from build123d import *

# Parameters (mm, degrees)
F0_W          = 57.15
F0_H          = 57.15
F0_W_2        = 51.054
F0_H_2        = 51.054
F1_DEPTH      = 304.8
F2_R          = 3.048
F3_R          = 6.35
F5_DEPTH      = 28.576
F5_DEPTH_BACK = 28.576
F7_DEPTH      = 28.576
F7_DEPTH_BACK = 28.576


with BuildPart() as f1:
    # F0 (on Top) → F1 (new body)
    with BuildSketch(Plane.XY):
        Rectangle(F0_W, F0_H)
        Rectangle(F0_W_2, F0_H_2, mode=Mode.SUBTRACT)
    extrude(amount=F1_DEPTH)

    # F2
    f2_edges = [f1.edges().sort_by_distance(p)[0] for p in [
        (25.527, 25.527, 152.4),
        (-25.527, 25.527, 152.4),
        (-25.527, -25.527, 152.4),
        (25.527, -25.527, 152.4),
    ]]
    fillet(f2_edges, radius=F2_R)

    # F3
    f3_edges = [f1.edges().sort_by_distance(p)[0] for p in [
        (-28.575, 28.575, 152.4),
        (-28.575, -28.575, 152.4),
        (28.575, -28.575, 152.4),
        (28.575, 28.575, 152.4),
    ]]
    fillet(f3_edges, radius=F3_R)

    # F4 (on Front) → F5 (cut, two sides)
    with BuildSketch(Plane.XZ) as f5_sk:
        Polygon((-28.575, 247.65), (28.575, 304.8), (-28.575, 304.8), align=None)
    extrude(amount=-F5_DEPTH, mode=Mode.SUBTRACT)
    extrude(f5_sk.sketch, amount=F5_DEPTH_BACK, mode=Mode.SUBTRACT)

    # F6 (on Front) → F7 (cut, two sides)
    with BuildSketch(Plane.XZ) as f7_sk:
        Polygon((28.575, 4.9999771205), (-28.575, 0), (28.575, 0), align=None)
    extrude(amount=-F7_DEPTH, mode=Mode.SUBTRACT)
    extrude(f7_sk.sketch, amount=F7_DEPTH_BACK, mode=Mode.SUBTRACT)


solid = f1.part
Work out the finished part from the listing and answer in its coordinate system (mm). A direction names the side the tool comes from. Give positions to 0.01 mm unless a question says otherwise; leave off trailing zeros. Order: outer loops, then holes, each group sorted by start corner. A loop starts at its lowest first (then second) coordinate and runs counter-clockwise, first axis right, second up. Notation, with made-up numbers: (-34.75, 5) -> (-21.75, 5) arc R12 cw to (-21.75, 27) -> close; hole circle Ø10 at (1.5, 5.25). An arc over 180 degrees is marked (long way). Answer as a JSON object with one key per item and string values. Group by question number.
1. A tool of negligible diameter and unlimited length cuts with its end or side. For faces 1 (the cylindrical face through (26.67, 26.76, 156.72)), 2 (the flat face through (0, -25.527, 148)), from which of +Z, -Z, +X, -X, +Y, -Y can it reach the whole face along a straight path? Write none if from no direction.
2. Section A-A on y = 1.5 is taken. Determine the outline of the cut face in (x, z) (3 decimals).
3. Section C-C on x = -14 is taken. Determine the outline of the cut face in (y, z) (3 decimals).
4. Section B-B on z = 223 is taken. Determine the outline of the cut face in (x, y) (3 decimals), plus the area to 3 significant figures.
5. The mould has two halves that part along Y. Classify faces 3 (the flat face through (-25.527, 0, 124)), 4 (the flat face through (-4.367, -27.65, 271.858)), 5 (the flat face through (0, 28.575, 147)): released by +Y, released by -Y, zero draft, split by the parting line, or undercut.
6. Section D-D on z = 273.5 is taken. Determine the outline of the cut face in (x, y) (3 decimals), plus the area to 3 significant figures.
7. Consider line 1 along Y through (x, z) = (-4.5, 21) (3 decimals); line 2 along X through (y, z) = (15, 263.5) (3 decimals). Determine where each line is inside the solid, lowest interval first. Write a range as [from, to].
8. A flat-ended cylindrical pin translates along its axis: pin 1 Ø8 at (y, z) = (22.5, 154.5) entering from -X (3 decimals). Find the tip coordinate at first contact, or state that the pin passes through.
Result sheet:
{
 "1": {"face 1": "+Z, -Z, +X, +Y", "face 2": "+Z, -Z"},
 "2": {"outline": "(-28.575, 0) -> (-25.527, 0.267) -> (-25.527, 250.698) -> (-28.575, 247.65) -> close; (25.527, 4.733) -> (28.575, 5) -> (28.575, 304.8) -> (25.527, 301.752) -> close"},
 "3": {"outline": "(-28.575, 1.275) -> (-25.527, 1.275) -> (-25.527, 262.225) -> (-28.575, 262.225) -> close; (25.527, 1.275) -> (28.575, 1.275) -> (28.575, 262.225) -> (25.527, 262.225) -> close"},
 "4": {"outline": "(-28.575, -22.225) arc R6.35 ccw to (-22.225, -28.575) -> (22.225, -28.575) arc R6.35 ccw to (28.575, -22.225) -> (28.575, 22.225) arc R6.35 ccw to (22.225, 28.575) -> (-22.225, 28.575) arc R6.35 ccw to (-28.575, 22.225) -> close; hole (-25.527, -22.479) arc R3.048 ccw to (-22.479, -25.527) -> (22.479, -25.527) arc R3.048 ccw to (25.527, -22.479) -> (25.527, 22.479) arc R3.048 ccw to (22.479, 25.527) -> (-22.479, 25.527) arc R3.048 ccw to (-25.527, 22.479) -> close", "area": "633 mm^2"},
 "5": {"face 3": "undercut", "face 4": "zero draft", "face 5": "released by +Y"},
 "6": {"outline": "(-2.725, -28.575) -> (22.225, -28.575) arc R6.35 ccw to (28.575, -22.225) -> (28.575, 22.225) arc R6.35 ccw to (22.225, 28.575) -> (-2.725, 28.575) -> (-2.725, 25.527) -> (22.479, 25.527) arc R3.048 cw to (25.527, 22.479) -> (25.527, -22.479) arc R3.048 cw to (22.479, -25.527) -> (-2.725, -25.527) -> close", "area": "333 mm^2"},
 "7": {"line 1": "y = [-28.575, -25.527], [25.527, 28.575]", "line 2": "x = [25.527, 28.575]"},
 "8": {"pin 1": "stops at x = -28.575"}
}
